Check sheet for the modelled part. Datum: model origin and axes. Units: mm. Face numbers are marked on the shaded views. A direction names the side the tool comes from. Give positions to 0.01 mm unless a question says otherwise; leave off trailing zeros. Order: outer loops, then holes, each group sorted by start corner. A loop starts at its lowest first (then second) coordinate and runs counter-clockwise, first axis right, second up.
Item 1: Sectioned sample at B-B on z = -1.75. Record the boundary of the cut face in (x, y).
Item 2: Access from +Z, -Z, +X, -X, +Y, -Y to the whole of each face (thin tool, end or side, straight path). Record for the marked faces 1, 2 and 3.
Item 3: Sectioned sample at A-A on y = -2.4. Count the separate pieces of the cut face and the enclosed holes in it, and give its area (3 significant figures).
Item 4: Gauge pin test, flat ends, axial feed: P1, Ø3, axis at x = 7, z = -1, coming from the +Y side; P2, Ø1, axis at x = 12, z = 1, coming from the +Y side. Record the tip position at first contact, or that the pin passes through.
Item 5: Material ranges on line 1 along Y through (x, z) = (11.25, -0.5); line 2 along X through (y, z) = (-1.2, 0); line 3 along Z through (x, y) = (13.75, -2.05), recorded low to high.
Item 6: Sectioned sample at C-C on x = 2. Record the boundary of the cut face in (y, z).
Item 7: Release check for a two-part mould opening along Z. For the marked faces 4, 5, 6 and 7 record: released by +Z, released by -Z, zero draft, split by the parting line, or undercut.
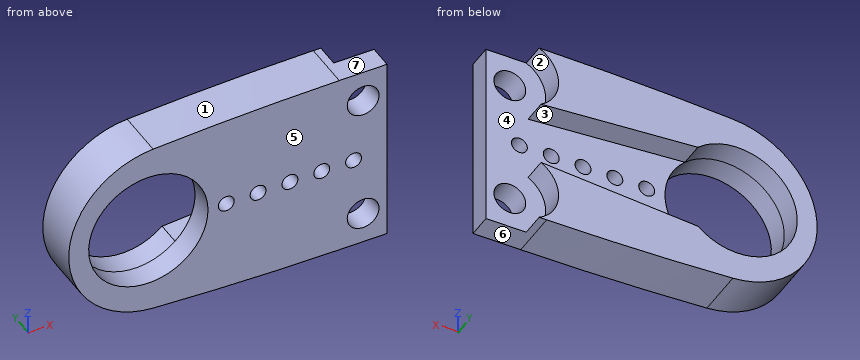
from build123d import *

# Parameters (mm, degrees)
SKETCH1_R               = 1
SKETCH1_R_2             = 2.35
BOSS_EXTRUDE1_DEPTH     = 3
ENL_V_MAT_EXTRU_1_DEPTH = 1.5
ESQUISSE3_R             = 0.5
ESQUISSE3_R_2           = 3.75
ENL_V_MAT_EXTRU_7_DEPTH = 17.224980878
ENL_V_MAT_EXTRU_8_DEPTH = 1.5


with BuildPart() as part:
    # Sketch1 → Boss-Extrude1 (new body)
    with BuildSketch(Plane(origin=(0, 0, 0), x_dir=(1, 0, 0), z_dir=(0, 1, 0))):
        with BuildLine():
            Line((15, 6), (12, 6))
            ThreePointArc((12, 6), (6.147204023, 5.909534011), (0.3, 5.638222479))
            ThreePointArc((0.3, 5.638222479), (-5, 0), (0.3, -5.638222479))
            ThreePointArc((0.3, -5.638222479), (6.147204023, -5.909534011), (12, -6))
            Line((12, -6), (15, -6))
            Line((15, -6), (15, 6))
        make_face()
        with Locations(Location((13.5, -4, 0), (0, 0, 270))):
            Circle(SKETCH1_R, mode=Mode.SUBTRACT)
        with Locations(Location((13.5, 4, 0), (0, 0, 270))):
            Circle(SKETCH1_R, mode=Mode.SUBTRACT)
        with Locations(Location((0, 0, 0), (0, 0, 270))):
            Circle(SKETCH1_R_2, mode=Mode.SUBTRACT)
    extrude(amount=-BOSS_EXTRUDE1_DEPTH)

    # Esquisse1 → Enlèv. mat.-Extru.1 (cut)
    with BuildSketch(Plane(origin=(0, 0, 0), x_dir=(1, 0, 0), z_dir=(0, 1, 0))):
        with BuildLine():
            Line((2.494493937, -2.8), (14.131406802, -1.932309126))
            add(Edge.make_bspline(
                [(14.131406802, -1.932309126), (14.497286128, -1.904835216), (14.827491954, -1.746052706), (15.157338026, -1.587443187), (15.407154881, -1.318584734), (15.656200737, -1.050556048), (15.790562016, -0.709168668), (15.92490372, -0.367831024), (15.925, 0), (15.925095847, 0.366175279), (15.791018176, 0.708007672), (15.657374187, 1.048734388), (15.407835717, 1.317851242), (15.159067388, 1.586137532), (14.828615817, 1.74551148), (14.498449498, 1.904747853), (14.131406802, 1.932309126)],
                knots=[0, 0, 0, 0.125, 0.125, 0.25, 0.25, 0.375, 0.375, 0.5, 0.5, 0.625, 0.625, 0.75, 0.75, 0.875, 0.875, 1, 1, 1], degree=2))
            Line((14.131406802, 1.932309126), (2.494493937, 2.8))
            ThreePointArc((2.494493937, 2.8), (-3.75, 0), (2.494493937, -2.8))
        make_face()
    extrude(amount=-ENL_V_MAT_EXTRU_1_DEPTH, mode=Mode.SUBTRACT)

    # Esquisse3 → Enlèv. mat.-Extru.7 (cut, through all)
    with BuildSketch(Plane(origin=(0, -1.5, 0), x_dir=(1, 0, 0), z_dir=(0, 1, 0))):
        with Locations(Location((4.9, 0, 0), (0, 0, 270))):
            Circle(ESQUISSE3_R)
        with Locations(Location((6.9, 0, 0), (0, 0, 270))):
            Circle(ESQUISSE3_R)
        with Locations(Location((8.9, 0, 0), (0, 0, 270))):
            Circle(ESQUISSE3_R)
        with Locations(Location((10.9, 0, 0), (0, 0, 270))):
            Circle(ESQUISSE3_R)
        with Locations(Location((12.9, 0, 0), (0, 0, 270))):
            Circle(ESQUISSE3_R)
        with Locations(Location((0, 0, 0), (0, 0, 270))):
            Circle(ESQUISSE3_R_2)
    extrude(amount=-ENL_V_MAT_EXTRU_7_DEPTH, mode=Mode.SUBTRACT)

    # Esquisse4 → Enlèv. mat.-Extru.8 (cut)
    with BuildSketch(Plane(origin=(0, 0, 0), x_dir=(1, 0, 0), z_dir=(0, 1, 0))):
        with BuildLine():
            Line((13.5, -1.75), (13.5, 1.75))
            ThreePointArc((13.5, 1.75), (11.25, 4), (13.5, 6.25))
            Line((13.5, 6.25), (13.5, 7.352249371))
            Line((13.5, 7.352249371), (16.575189436, 7.352249371))
            Line((16.575189436, 7.352249371), (16.575189436, -9.01785128))
            Line((16.575189436, -9.01785128), (13.5, -9.01785128))
            Line((13.5, -9.01785128), (13.5, -6.25))
            ThreePointArc((13.5, -6.25), (11.25, -4), (13.5, -1.75))
        make_face()
    extrude(amount=-ENL_V_MAT_EXTRU_8_DEPTH, mode=Mode.SUBTRACT)


solid = part.part
Report:
1. outline: (-4.72, -3) - (-3.32, -3) - (-3.32, 0) - (-4.72, 0) - close; (3.32, -3) - (15, -3) - (15, -1.5) - (3.32, -1.5) - close
2. face 1: +Z, -X, +Y, -Y
2. face 2: +X, +Y
2. face 3: +Y
3. separate pieces: 1
3. enclosed holes: 8
3. area: 165 mm2
4. P1: stops at y = 0
4. P2: stops at y = -1.5
5. line 1: y = -3 to -1.5
5. line 2: x = -5 to -3.75
5. line 3: z = -6 to -4.97, -3.03 to 3.03, 4.97 to 6
6. outline: (-3, -5.74) - (0, -5.74) - (0, -3.17) - (-3, -3.17) - close; (-3, 3.17) - (0, 3.17) - (0, 5.74) - (-3, 5.74) - close
7. face 4: undercut
7. face 5: zero draft
7. face 6: released by -Z
7. face 7: released by +Z
